Autodesk Inventor part; units mm, degrees
ref_plane "YZ Plane" through (0, 0, 0) normal (1, 0, 0) x (0, 1, 0)
ref_plane "XZ Plane" through (0, 0, 0) normal (0, 1, 0) x (-1, 0, 0)
ref_plane "XY Plane" through (0, 0, 0) normal (0, 0, 1) x (1, 0, 0)
sketch "Sketch1" plane through (0, 0, 0) normal (0, 0, 1) x (1, 0, 0)
  line L0 (9.7751, 75.6011) -> (11.7751, 75.6011)
  line L1 (52.7751, 75.6011) -> (54.7751, 75.6011)
  arc A0 (22.5579, 17.6142) -> (42.1677, 17.6615) centre (32.3508, 22.6241) ccw
  line L2 (9.7751, 42.6011) -> (54.7751, 42.6011)
  line L3 (11.7751, 44.6011) -> (52.7751, 44.6011)
  line L4 (11.7751, 75.6011) -> (11.7751, 44.6011)
  line L5 (9.7751, 75.6011) -> (9.7751, 42.6011)
  line L6 (52.7751, 75.6011) -> (52.7751, 44.6011)
  line L7 (54.7751, 75.6011) -> (54.7751, 42.6011)
  line L8 (54.7751, 42.6011) -> (42.1677, 17.6615)
  line L9 (9.7751, 42.6011) -> (22.5579, 17.6142)
  circle A1 centre (32.3508, 22.6241) radius 4.5
  point P0 (0, 0)
  dimension "d15" = 9
extrude "Extrusion1" add sketch "Sketch1" against normal blind 45
sketch "Sketch2" plane through (54.7751, 42.6011, 0) normal (1, 0, 0) x (0, 0, -1)
  circle A0 centre (22.5, 22) radius 11
  line L0 (0, 0) -> (0, 2)
  line L1 (0, 33) -> (0, 0)
  line L2 (45, 0) -> (45, 2)
  line L3 (45, 33) -> (45, 0)
  line L4 (45, 2) -> (32.3068, 26.9826)
  line L5 (0, 2) -> (12.6932, 26.9826)
  line L6 (0, 2) -> (0, 38)
  line L7 (0, 38) -> (45, 38)
  line L8 (45, 38) -> (45, 2)
  circle A1 centre (22.5, 22) radius 4.5
  line L9 (0, 0) -> (45, 0)
  line L10 (45, -24.9396) -> (45, 0)
  point P0 (0, -42.6011)
  dimension "d2" = 22
  dimension "d16" = 9
extrude "Extrusion2" cut sketch "Sketch2" against normal blind 45 contours A0 L5 L1 L6 L7 L8 L3 L4 | A1
sketch "Sketch3" plane through (54.7751, 42.6011, 0) normal (1, 0, 0) x (0, 0, -1)
  line L0 (0, 0) -> (45, 0)
  line L1 (43, 0) -> (2, 0)
  line L2 (2, 0) -> (2, -33)
  line L3 (2, -33) -> (43, -33)
  line L4 (43, -33) -> (43, 0)
  line L5 (45, -24.9396) -> (45, 0)
  point P0 (0, -42.6011)
  dimension "d9" = 41
  dimension "d10" = 2
extrude "Extrusion3" cut sketch "Sketch3" against normal blind 45
sketch "Sketch5" plane through (0, 0, 0) normal (0, 0, 1) x (1, 0, 0)
  line L0 (9.7751, 42.6011) -> (22.5579, 17.6142)
  arc A0 (22.5579, 17.6142) -> (42.1677, 17.6615) centre (32.3508, 22.6241) ccw
  line L1 (42.1677, 17.6615) -> (54.7751, 42.6011)
  line L2 (52.7751, 44.6011) -> (11.7751, 44.6011)
  circle A1 centre (32.3508, 22.6241) radius 4.5
  line L3 (27.8508, 22.6241) -> (27.8508, 12.5867)
  line L4 (36.8508, 22.6241) -> (36.8508, 12.5867)
  arc A2 (36.8508, 22.6241) -> (27.8508, 22.6241) centre (32.3508, 22.6241) ccw
  arc A3 (27.8508, 12.5867) -> (36.8508, 12.5867) centre (32.3508, 22.6241) ccw
  point P0 (0, 0)
extrude "Extrusion4" cut sketch "Sketch5" against normal through all
sketch "Sketch6" plane through (54.7751, 42.6011, 0) normal (1, 0, 0) x (0, 0, -1)
  arc A0 (32.3068, 26.9826) -> (12.6932, 26.9826) centre (22.5, 22) ccw
  arc A1 (18, 22) -> (27, 22) centre (22.5, 22) ccw
  line L0 (18, 22) -> (18, 34.9118)
  line L1 (27, 22) -> (27, 34.9118)
  line L2 (27, 34.9118) -> (18, 34.9118)
  point P0 (0, -42.6011)
  dimension "d19" = 9
extrude "Extrusion5" cut sketch "Sketch6" against normal through all
sketch "Sketch7" plane through (0, 0, -45) normal (0, 0, -1) x (-1, 0, 0)
  arc A0 (-27.8508, 12.5867) -> (-22.5579, 17.6142) centre (-32.3508, 22.6241) ccw
  circle A1 centre (-24.4978, 25.8769) radius 1
  point P0 (0, 0)
  dimension "d22" = 2
  dimension "d23" = 8.5
extrude "Extrusion6" cut sketch "Sketch7" against normal through all
pattern_circular "Circular Pattern1" count 8 over 360 about axis through (32.3508, 22.6241, 0) along (0, 0, -1) of "Extrusion6"
sketch "Sketch8" plane through (9.7751, 42.6011, 0) normal (-1, 0, 0) x (0, 0, 1)
  arc A0 (-27, 22) -> (-18, 22) centre (-22.5, 22) ccw
  line L0 (-22.5, 22) -> (-14.647, 25.2528)
  line L1 (-22.5, 22) -> (-14, 22) construction
  circle A1 centre (-14.647, 25.2528) radius 1
  point P0 (0, -42.6011)
  dimension "d29" = 8.5
  dimension "d30" = 22.5
  dimension "d31" = 2
extrude "Extrusion7" cut sketch "Sketch8" against normal through all
pattern_circular "Circular Pattern2" count 8 over 360 about axis through (54.7751, 64.6011, -22.5) along (-1, 0, 0) of "Extrusion7"
properties part number "Ankle" material "Aluminum-6061"
Part model, mm, in its own coordinate system. A direction names the side the tool comes from. Round coordinates to 2 decimals unless told otherwise and drop trailing zeros. Write each loop counter-clockwise with the first axis right and the second up, starting at its lowest first coordinate (ties: lowest second). Pieces come first, ordered by that corner, then holes. Notation, with made-up numbers: M 89.25,49.25 L 96.25,49.25 A33 ccw 96.25,82.25 Z; hole C 21.5,57 d9. An arc over 180 degrees is marked long. Answer as CSV lines item,"result". Start each with the question number.
1) Drop flat-ended pins along their axis: pin 1 (1.2 mm diameter, centred on y = 56.75, z = -19.25, fed in from +X); pin 2 (8 mm diameter, centred on x = 16, z = -18.5, fed in from +Y); pin 3 (2 mm diameter, centred on x = 39, z = -6.5, fed in from -Y); pin 4 (1 mm diameter, centred on y = 19, z = -1.5, fed in from -X). Give the stop position or say it passes through.
2) Mould opens along X. For faces 1 (the face through (29.314, 31.453, -44.014)), 2 (the face through (10.761, 60.424, -14.265)), 3 (the face through (48.56, 30.31, -0.99)) say: +X half, -X half, draft (parallel to the pull), parting line (faces both ways), or undercut.
3) Band-saw the part on A-A (z = -22.5). List the corners of the cut face in (x, y).
4) Band-saw the part on B-B (x = 31). List the corners of the cut face in (y, z).
5) Which spindle directions (+Z, -Z, +X, -X, +Y, -Y) get a long thin tool onto all of the face, cutting with end or side? Do faces 4 (the face through (10.79, 72.6, -14.95)), 5 (the face through (36.851, 18, -1)), 6 (the face through (54, 70, -18)). Say none if no direction does.
6) Drill centre lines: L1, parallel to Z at x = 25.5, y = 32.5; L2, parallel to X at y = 59, z = -8; L3, parallel to Y at x = 20.5, z = -27. Where is each one in solid material? Low to high.
Worked out:
1,pin 1,"through"
1,pin 2,"y = 44.6"
1,pin 3,"y = 42.6"
1,pin 4,"x = 21.59"
2,face 1,"undercut"
2,face 2,"draft"
2,face 3,"+X half"
3,outline,"M 9.78,42.6 L 54.78,42.6 L 54.78,60.1 L 52.78,60.1 L 52.78,44.6 L 11.78,44.6 L 11.78,60.1 L 9.78,60.1 Z"
4,outline,"M 26.92,-45 L 44.6,-45 L 44.6,0 L 26.92,0 L 26.92,-2 L 42.6,-2 L 42.6,-43 L 26.92,-43 Z"
5,face 4,"+Z, +X, -X, +Y"
5,face 5,"+Z, -Z, -Y"
5,face 6,"+X, -X, +Y"
6,L1,"-45 to -43, -2 to 0"
6,L2,"9.78 to 11.78, 52.78 to 54.78"
6,L3,"42.6 to 44.6"
